Could you check a few things on this model? Use its own coordinates, in mm. Coordinates: 2 decimals unless noted, no trailing zeros. Loops run counter-clockwise (first coordinate to the right, second up) from the corner with the lowest first, then second, coordinate; pieces in that order, holes last.
1) If I drill on line 1 along Y through (x, z) = (-9.75, 0.3); line 2 along X through (y, z) = (7.5, 0.4); line 3 along Y through (x, z) = (-9.5, 0.4), over which ranges is the centre line in solid material (lowest first)?
2) Imagine slicing it at A-A on z = 0.1. Please give me the cut outline in (x, y), plus the area to 3 significant figures.
3) Imagine slicing it at B-B on y = -5.25. Please give me the cut outline in (x, z), plus the area to 3 significant figures.
4) Imagine slicing it at C-C on x = -9.75. Please give me the cut outline in (y, z), plus the area to 3 significant figures.
```python
from build123d import *

# Parameters (mm, degrees)
F1_DEPTH = 0.5
F3_DEPTH = 0.501


with BuildPart() as f1:
    # F0 (on Top) → F1 (new body)
    with BuildSketch(Plane.XY):
        Polygon((6.25, -10.825318), (12.5, 0), (6.25, 10.825318), (-6.25, 10.825318), (-12.5, 0), (-6.25, -10.825318), align=None)
    extrude(amount=F1_DEPTH)

    # F2 (on face) → F3 (cut, through all)
    with BuildSketch(Plane.XY.offset(0.5)):
        with BuildLine():
            ThreePointArc((0.85, -10.825318), (0.674264, -10.401053), (0.25, -10.225318))
            Line((0.25, -10.225318), (-0.25, -10.225318))
            ThreePointArc((-0.25, -10.225318), (-0.674264, -10.401053), (-0.85, -10.825318))
            Line((-0.85, -10.825318), (0.85, -10.825318))
        make_face()
    extrude(amount=-F3_DEPTH, mode=Mode.SUBTRACT)


solid = f1.part
```
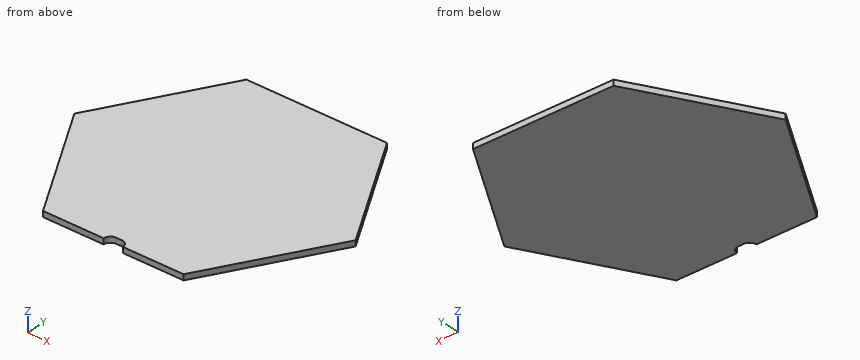
Filled in:
1. line 1: y = -4.76 to 4.76
1. line 2: x = -8.17 to 8.17
1. line 3: y = -5.2 to 5.2
2. outline: (-12.5, 0) - (-6.25, -10.83) - (-0.85, -10.83) arc R0.6 cw to (-0.25, -10.23) - (0.25, -10.23) arc R0.6 cw to (0.85, -10.83) - (6.25, -10.83) - (12.5, 0) - (6.25, 10.83) - (-6.25, 10.83) - close
2. area: 405 mm2
3. outline: (-9.47, 0) - (9.47, 0) - (9.47, 0.5) - (-9.47, 0.5) - close
3. area: 9.47 mm2
4. outline: (-4.76, 0) - (4.76, 0) - (4.76, 0.5) - (-4.76, 0.5) - close
4. area: 4.76 mm2
